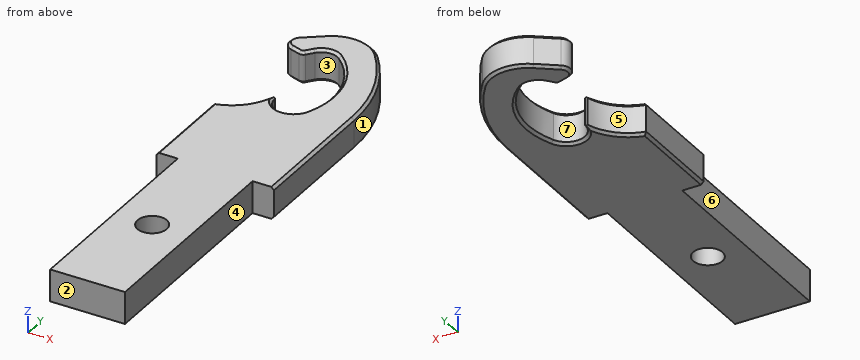
```python
from build123d import *

# Parameters (mm, degrees)
SKETCH_1_R      = 27.5
EXTRUDE_1_DEPTH = 30
CHAMFER_1_SIZE  = 5


with BuildPart() as part:
    # 草图1 → 凸台-拉伸1 (new, symmetric)
    with BuildSketch(Plane.XY):
        with BuildLine():
            Line((140, 405), (180, 405))
            Line((180, 405), (180, 659.74236495))
            ThreePointArc((180, 659.74236495), (162.31188427, 761.231280601), (111.333333333, 850.752545017))
            ThreePointArc((111.333333333, 850.752545017), (62.369816768, 877.473662126), (8.5, 863))
            Line((8.5, 863), (-27.5, 836))
            ThreePointArc((-27.5, 836), (-35.196294357, 816.527826528), (-21.305524623, 800.861142044))
            Line((-21.305524623, 800.861142044), (-3.402762311, 795.430571022))
            ThreePointArc((-3.402762311, 795.430571022), (2.420792013, 795.436058657), (7.253794336, 798.685043674))
            Line((7.253794336, 798.685043674), (17.238616993, 810.944868978))
            ThreePointArc((17.238616993, 810.944868978), (37.541078237, 821.853723084), (59.589937945, 815.142477595))
            ThreePointArc((59.589937945, 815.142477595), (109.84673197, 735.06182538), (102.218185324, 640.825624899))
            ThreePointArc((102.218185324, 640.825624899), (63.022768685, 620.202503835), (35, 654.5))
            Line((35, 654.5), (30.481942633, 654.5))
            ThreePointArc((30.481942633, 654.5), (4.791252117, 610.80152605), (-40, 587.067332603))
            Line((-40, 587.067332603), (-40, 405))
            Line((-40, 405), (0, 405))
            Line((0, 405), (0, 0))
            Line((0, 0), (140, 0))
            Line((140, 0), (140, 405))
        make_face()
        with Locations((70, 205)):
            Circle(SKETCH_1_R, mode=Mode.SUBTRACT)
    extrude(amount=EXTRUDE_1_DEPTH, both=True)

    # 倒角1
    # the kernel refuses this chamfer: 5 mm, written as the material it takes off along each edge
    with BuildSketch(Plane(origin=(-59.5, 678, -30), x_dir=(0.9931437230377144, -0.11689972365573639, 0), z_dir=(0.11689972365573639, 0.9931437230377144, 0))) as chamfer_1_piece_1:
        Polygon((93, -CHAMFER_1_SIZE), (93 + CHAMFER_1_SIZE, 0), (93, 0), align=None)
    revolve(axis=Axis((-59.5, 678, -30), (0, 0, -1)), revolution_arc=79.106771972, mode=Mode.SUBTRACT)
    with BuildSketch(Plane(origin=(-59.5, 678, 30), x_dir=(0.9931437230377144, -0.11689972365573639, 0), z_dir=(0.11689972365573639, 0.9931437230377144, 0))) as chamfer_1_piece_2:
        Polygon((93 + CHAMFER_1_SIZE, 0), (93, CHAMFER_1_SIZE), (93, 0), align=None)
    revolve(axis=Axis((-59.5, 678, 30), (0, 0, -1)), revolution_arc=79.106771972, mode=Mode.SUBTRACT)
    with BuildSketch(Plane(origin=(180, 392.14158506, -30), x_dir=(0.0274958766105877, 0, 0.9996219169112968), z_dir=(0, 1, 0))) as chamfer_1_piece_3:
        Polygon((CHAMFER_1_SIZE * 0.999621916911, -CHAMFER_1_SIZE * 0.0274958766106), (-CHAMFER_1_SIZE * 0.0274958766106, -CHAMFER_1_SIZE * 0.999621916911), (0, 0), align=None)
    extrude(amount=267.60077989, mode=Mode.SUBTRACT)
    with BuildSketch(Plane(origin=(-120, 659.74236495, -30), x_dir=(1, 0, 0), z_dir=(0, -1, 0))) as chamfer_1_piece_4:
        Polygon((300, CHAMFER_1_SIZE), (300 - CHAMFER_1_SIZE, 0), (300, 0), align=None)
    revolve(axis=Axis((-120, 659.74236495, -30), (0, 0, 1)), revolution_arc=39.546229231, mode=Mode.SUBTRACT)
    with BuildSketch(Plane(origin=(53.5, 803, -30), x_dir=(0.7711111111111113, 0.6367006002203762, 0), z_dir=(0.6367006002203762, -0.7711111111111113, 0))) as chamfer_1_piece_5:
        Polygon((75, CHAMFER_1_SIZE), (75 - CHAMFER_1_SIZE, 0), (75, 0), align=None)
    revolve(axis=Axis((53.5, 803, -30), (0, 0, 1)), revolution_arc=87.323668415, mode=Mode.SUBTRACT)
    with BuildSketch(Plane(origin=(8.5, 863, -30), x_dir=(-0.01649752596635013, 0.02199670128846693, 0.9996219169112968), z_dir=(-0.8000000000000013, -0.5999999999999984, 0))) as chamfer_1_piece_6:
        Polygon((CHAMFER_1_SIZE * 0.999621916911, -CHAMFER_1_SIZE * 0.0274958766106), (-CHAMFER_1_SIZE * 0.0274958766106, -CHAMFER_1_SIZE * 0.999621916911), (0, 0), align=None)
    extrude(amount=45, mode=Mode.SUBTRACT)
    with BuildSketch(Plane(origin=(-15.5, 820, -30), x_dir=(-0.6000000000000103, 0.7999999999999922, 0), z_dir=(0.7999999999999922, 0.6000000000000103, 0))) as chamfer_1_piece_7:
        Polygon((20, CHAMFER_1_SIZE), (20 - CHAMFER_1_SIZE, 0), (20, 0), align=None)
    revolve(axis=Axis((-15.5, 820, -30), (0, 0, 1)), revolution_arc=126.255608056, mode=Mode.SUBTRACT)
    with BuildSketch(Plane(origin=(-21.305524623, 800.861142044, -30), x_dir=(-0.007981399434105696, -0.02631198384115636, 0.9996219169112971), z_dir=(0.9569428977956573, -0.29027623112898887, 0))) as chamfer_1_piece_8:
        Polygon((CHAMFER_1_SIZE * 0.999621916911, -CHAMFER_1_SIZE * 0.0274958766106), (-CHAMFER_1_SIZE * 0.0274958766106, -CHAMFER_1_SIZE * 0.999621916911), (0, 0), align=None)
    extrude(amount=18.708286934, mode=Mode.SUBTRACT)
    with BuildSketch(Plane(origin=(-0.5, 805, -30), x_dir=(-0.29027623112897577, -0.9569428977956612, 0), z_dir=(-0.9569428977956612, 0.29027623112897577, 0))) as chamfer_1_piece_9:
        Polygon((10, CHAMFER_1_SIZE), (10 - CHAMFER_1_SIZE, 0), (10, 0), align=None)
    revolve(axis=Axis((-0.5, 805, -30), (0, 0, 1)), revolution_arc=67.7139403, mode=Mode.SUBTRACT)
    with BuildSketch(Plane(origin=(7.253794336, 798.685043674, -30), x_dir=(0.021319737231601184, -0.01736352599446127, 0.9996219169112965), z_dir=(0.6314956326132553, 0.7753794335616496, 0))) as chamfer_1_piece_10:
        Polygon((CHAMFER_1_SIZE * 0.999621916911, -CHAMFER_1_SIZE * 0.0274958766106), (-CHAMFER_1_SIZE * 0.0274958766106, -CHAMFER_1_SIZE * 0.999621916911), (0, 0), align=None)
    extrude(amount=15.811388301, mode=Mode.SUBTRACT)
    with BuildSketch(Plane(origin=(40.5, 792, -30), x_dir=(-0.7753794335616501, 0.6314956326132546, 0), z_dir=(-0.6314956326132546, -0.7753794335616501, 0))) as chamfer_1_piece_11:
        Polygon((30, -CHAMFER_1_SIZE), (30 + CHAMFER_1_SIZE, 0), (30, 0), align=None)
    revolve(axis=Axis((40.5, 792, -30), (0, 0, -1)), revolution_arc=90.358237971, mode=Mode.SUBTRACT)
    with BuildSketch(Plane(origin=(-35.85975178, 699.430089618, -30), x_dir=(0.6363312648327024, 0.7714159198489573, 0), z_dir=(-0.7714159198489573, 0.6363312648327024, 0))) as chamfer_1_piece_12:
        Polygon((150, -CHAMFER_1_SIZE), (150 + CHAMFER_1_SIZE, 0), (150, 0), align=None)
    revolve(axis=Axis((-35.85975178, 699.430089618, -30), (0, 0, -1)), revolution_arc=73.479048371, mode=Mode.SUBTRACT)
    with BuildSketch(Plane(origin=(70, 654.5, -30), x_dir=(0.920519580694994, -0.39069643146196303, 0), z_dir=(0.39069643146196303, 0.920519580694994, 0))) as chamfer_1_piece_13:
        Polygon((35, -CHAMFER_1_SIZE), (35 + CHAMFER_1_SIZE, 0), (35, 0), align=None)
    revolve(axis=Axis((70, 654.5, -30), (0, 0, -1)), revolution_arc=178.077418405, mode=Mode.SUBTRACT)
    with BuildSketch(Plane(origin=(180, 392.14158506, 30), x_dir=(0.0274958766105877, 0, -0.9996219169112968), z_dir=(0, 1, 0))) as chamfer_1_piece_14:
        Polygon((CHAMFER_1_SIZE * 0.999621916911, CHAMFER_1_SIZE * 0.0274958766106), (-CHAMFER_1_SIZE * 0.0274958766106, CHAMFER_1_SIZE * 0.999621916911), (0, 0), align=None)
    extrude(amount=267.60077989, mode=Mode.SUBTRACT)
    with BuildSketch(Plane(origin=(-120, 659.74236495, 30), x_dir=(1, 0, 0), z_dir=(0, -1, 0))) as chamfer_1_piece_15:
        Polygon((300, -CHAMFER_1_SIZE), (300 - CHAMFER_1_SIZE, 0), (300, 0), align=None)
    revolve(axis=Axis((-120, 659.74236495, 30), (0, 0, 1)), revolution_arc=39.546229231, mode=Mode.SUBTRACT)
    with BuildSketch(Plane(origin=(53.5, 803, 30), x_dir=(0.7711111111111113, 0.6367006002203762, 0), z_dir=(0.6367006002203762, -0.7711111111111113, 0))) as chamfer_1_piece_16:
        Polygon((75, -CHAMFER_1_SIZE), (75 - CHAMFER_1_SIZE, 0), (75, 0), align=None)
    revolve(axis=Axis((53.5, 803, 30), (0, 0, 1)), revolution_arc=87.323668415, mode=Mode.SUBTRACT)
    with BuildSketch(Plane(origin=(8.5, 863, 30), x_dir=(-0.01649752596635013, 0.02199670128846693, -0.9996219169112968), z_dir=(-0.8000000000000013, -0.5999999999999984, 0))) as chamfer_1_piece_17:
        Polygon((CHAMFER_1_SIZE * 0.999621916911, CHAMFER_1_SIZE * 0.0274958766106), (-CHAMFER_1_SIZE * 0.0274958766106, CHAMFER_1_SIZE * 0.999621916911), (0, 0), align=None)
    extrude(amount=45, mode=Mode.SUBTRACT)
    with BuildSketch(Plane(origin=(-15.5, 820, 30), x_dir=(-0.6000000000000103, 0.7999999999999922, 0), z_dir=(0.7999999999999922, 0.6000000000000103, 0))) as chamfer_1_piece_18:
        Polygon((20, -CHAMFER_1_SIZE), (20 - CHAMFER_1_SIZE, 0), (20, 0), align=None)
    revolve(axis=Axis((-15.5, 820, 30), (0, 0, 1)), revolution_arc=126.255608056, mode=Mode.SUBTRACT)
    with BuildSketch(Plane(origin=(-21.305524623, 800.861142044, 30), x_dir=(-0.007981399434105696, -0.02631198384115636, -0.9996219169112971), z_dir=(0.9569428977956573, -0.29027623112898887, 0))) as chamfer_1_piece_19:
        Polygon((CHAMFER_1_SIZE * 0.999621916911, CHAMFER_1_SIZE * 0.0274958766106), (-CHAMFER_1_SIZE * 0.0274958766106, CHAMFER_1_SIZE * 0.999621916911), (0, 0), align=None)
    extrude(amount=18.708286934, mode=Mode.SUBTRACT)
    with BuildSketch(Plane(origin=(-0.5, 805, 30), x_dir=(-0.29027623112897577, -0.9569428977956612, 0), z_dir=(-0.9569428977956612, 0.29027623112897577, 0))) as chamfer_1_piece_20:
        Polygon((10, -CHAMFER_1_SIZE), (10 - CHAMFER_1_SIZE, 0), (10, 0), align=None)
    revolve(axis=Axis((-0.5, 805, 30), (0, 0, 1)), revolution_arc=67.7139403, mode=Mode.SUBTRACT)
    with BuildSketch(Plane(origin=(7.253794336, 798.685043674, 30), x_dir=(0.021319737231601184, -0.01736352599446127, -0.9996219169112965), z_dir=(0.6314956326132553, 0.7753794335616496, 0))) as chamfer_1_piece_21:
        Polygon((CHAMFER_1_SIZE * 0.999621916911, CHAMFER_1_SIZE * 0.0274958766106), (-CHAMFER_1_SIZE * 0.0274958766106, CHAMFER_1_SIZE * 0.999621916911), (0, 0), align=None)
    extrude(amount=15.811388301, mode=Mode.SUBTRACT)
    with BuildSketch(Plane(origin=(40.5, 792, 30), x_dir=(-0.7753794335616501, 0.6314956326132546, 0), z_dir=(-0.6314956326132546, -0.7753794335616501, 0))) as chamfer_1_piece_22:
        Polygon((30, CHAMFER_1_SIZE), (30 + CHAMFER_1_SIZE, 0), (30, 0), align=None)
    revolve(axis=Axis((40.5, 792, 30), (0, 0, -1)), revolution_arc=90.358237971, mode=Mode.SUBTRACT)
    with BuildSketch(Plane(origin=(-35.85975178, 699.430089618, 30), x_dir=(0.6363312648327024, 0.7714159198489573, 0), z_dir=(-0.7714159198489573, 0.6363312648327024, 0))) as chamfer_1_piece_23:
        Polygon((150, CHAMFER_1_SIZE), (150 + CHAMFER_1_SIZE, 0), (150, 0), align=None)
    revolve(axis=Axis((-35.85975178, 699.430089618, 30), (0, 0, -1)), revolution_arc=73.479048371, mode=Mode.SUBTRACT)
    with BuildSketch(Plane(origin=(70, 654.5, 30), x_dir=(0.920519580694994, -0.39069643146196303, 0), z_dir=(0.39069643146196303, 0.920519580694994, 0))) as chamfer_1_piece_24:
        Polygon((35, CHAMFER_1_SIZE), (35 + CHAMFER_1_SIZE, 0), (35, 0), align=None)
    revolve(axis=Axis((70, 654.5, 30), (0, 0, -1)), revolution_arc=178.077418405, mode=Mode.SUBTRACT)
    with BuildSketch(Plane(origin=(-40, 599.925747542, -30), x_dir=(-0.027495876610586317, 0, 0.9996219169112968), z_dir=(0, -1, 0))) as chamfer_1_piece_25:
        Polygon((CHAMFER_1_SIZE * 0.999621916911, -CHAMFER_1_SIZE * 0.0274958766106), (-CHAMFER_1_SIZE * 0.0274958766106, -CHAMFER_1_SIZE * 0.999621916911), (0, 0), align=None)
    extrude(amount=207.784162482, mode=Mode.SUBTRACT)
    with BuildSketch(Plane(origin=(-40, 599.925747542, 30), x_dir=(-0.027495876610586317, 0, -0.9996219169112968), z_dir=(0, -1, 0))) as chamfer_1_piece_26:
        Polygon((CHAMFER_1_SIZE * 0.999621916911, CHAMFER_1_SIZE * 0.0274958766106), (-CHAMFER_1_SIZE * 0.0274958766106, CHAMFER_1_SIZE * 0.999621916911), (0, 0), align=None)
    extrude(amount=207.784162482, mode=Mode.SUBTRACT)


solid = part.part
```
Here's how the part is built. I have some questions about the finished solid (model axes, mm). Face numbers are marked on the shaded views. A direction names the side the tool comes from. Give positions to 0.01 mm unless a question says otherwise; leave off trailing zeros. Loops run counter-clockwise (first coordinate to the right, second up) from the corner with the lowest first, then second, coordinate; pieces in that order, holes last. Notation, with made-up numbers: M 14,13.25 L 65,13.25 A19 cw 65,17.25 Z; hole C 9,69.25 d7. An arc over 180 degrees is marked long. Return JSON: item names as keys, results as strings.
Item 1: Thinking about a two-plate mould opening in X: for the marked faces 1, 2 and 3, which applies, released by +X, released by -X, zero draft, split by the parting line, or undercut?
A:
{"face 1": "released by +X", "face 2": "zero draft", "face 3": "undercut"}
Item 2: I'm going to push flat-ended pins straight in: pin 1 Ø2.5 at (x, z) = (32, 6.5) entering from +Y; pin 2 Ø2 at (y, z) = (717, 10) entering from -X; pin 3 Ø8 at (y, z) = (230.5, -21.5) entering from +X. Where does each tip first touch, or does it pass through?
A:
{"pin 1": "stops at y = 875.21", "pin 2": "stops at x = 112.99", "pin 3": "stops at x = 140"}
Item 3: Please list where these lines run through material, in increasing order: line 1 (Y direction, x = 70, z = 6.5); line 2 (Y direction, x = 63, z = 7); line 3 (Y direction, x = 16.5, z = -9).
A:
{"line 1": "y = 0 to 177.5, 232.5 to 619.5, 805.7 to 876.16", "line 2": "y = 0 to 178.41, 231.59 to 620.21, 812.24 to 877.4", "line 3": "y = 0 to 624.4, 810.04 to 868.24"}
Item 4: Imagine slicing it at A-A on y = 205. List the corners of the cut face in (x, z) for me, then the cut area to 3 significant figures.
A:
{"outline": "M 0,-30 L 42.5,-30 L 42.5,30 L 0,30 Z; M 97.5,-30 L 140,-30 L 140,30 L 97.5,30 Z", "area": "5,100 mm^2"}
Item 5: Imagine slicing it at B-B on z = 17. List the corners of the cut face in (x, y) for me, then the cut area to 3 significant figures.
A:
{"outline": "M -40,405 L 0,405 L 0,0 L 140,0 L 140,405 L 180,405 L 180,659.74 A300 ccw 111.33,850.75 A75 ccw 8.5,863 L -27.5,836 A20 ccw -21.31,800.86 L -3.4,795.43 A10 ccw 7.25,798.69 L 17.24,810.94 A30 cw 59.59,815.14 A150 cw 102.22,640.83 A35 cw 35,654.5 L 30.48,654.5 A93 cw -40,587.07 Z; hole C 70,205 d55", "area": "123,000 mm^2"}
Item 6: On a 3-axis mill with a long thin cutter (end or side, diameter ignored), from which of +Z, -Z, +X, -X, +Y, -Y can I reach the whole of each face in a straight line? I mean the marked faces 4, 5, 6 and 7. Say none if no direction works.
A:
{"face 4": "+Z, -Z, +X, -Y", "face 5": "+Z, -Z, -X", "face 6": "+Z, -Z, -X, -Y", "face 7": "+Z, -Z"}
